```python
from build123d import *

# Parameters (mm, degrees)
F0_R     = 500
F2_DEPTH = 25
F1_R     = 46.69
F3_DEPTH = 300
F4_COUNT = 5


with BuildPart() as f2:
    # F0 (on Top) → F2 (new body)
    with BuildSketch(Plane.XY):
        Circle(F0_R)
    extrude(amount=F2_DEPTH)

    # F1 (on face) → F3 (join)
    with BuildSketch(Plane.XY):
        with Locations((0, -403.2496213913)):
            Circle(F1_R)
    extrude(amount=-F3_DEPTH)

    # F4: F2 ×5 about axis
    f4_axis = Axis((0, 0, 0), (0, 0, 1))


with BuildPart() as f2_1:
    add(f2.part)
    for i in range(1, F4_COUNT):
        add(f2.part.rotate(f4_axis, i * 360 / F4_COUNT))


solid = f2_1.part
```
Work out the finished part from the listing and answer in its coordinate system (mm). A direction names the side the tool comes from. Round coordinates to 2 decimals unless told otherwise and drop trailing zeros. Write each loop counter-clockwise with the first axis right and the second up, starting at its lowest first coordinate (ties: lowest second). Pieces come first, ordered by that corner, then holes.
1) A cutting plane is placed at A-A on x = 0. Determine the outline of the cut face in (y, z).
2) A cutting plane is placed at D-D on x = -219.5. Determine the outline of the cut face in (y, z).
3) Flat-ended cylindrical pins translate along their axes: P1, Ø12, axis at y = -90.5, z = -157, coming from the +X side; P2, Ø5, axis at x = -304, y = 112, coming from the -Z side; P3, Ø10, axis at x = -204.5, z = -213.5, coming from the +Y side. Find the tip coordinate at first contact, or state that the pin passes through.
4) A cutting plane is placed at B-B on z = -151. Determine the outline of the cut face in (x, y), and give its area (3 significant figures).
5) Which of the six approach directions +Z, -Z, +X, -X, +Y, -Y give full straight-line access (tool end or side, diameter ignored) to faces 5 (the face through (-7, 7, 0)), 6 (the face through (-236, 326, -300))?
6) A cutting plane is placed at C-C on y = 0. Determine the outline of the cut face in (x, z), and give its area (3 significant figures).
7) Consider probe 1 along Z at (x, y) = (198, -176.5); probe 2 along X at (y, z) = (-99.5, -115.5); probe 3 along X at (y, z) = (368, -97). Determine where each line is inside the solid, lowest interval first.
8) Determine the mould class of faces 1 (the face through (-383, -124, -300)), 2 (the face through (214.731, 285.212, -147.9)), 3 (the face through (383.937, -77.923, -147.9)), 4 (the face through (21.545, -444.672, -147.9)) for opening direction X: pulls with the +X half, pulls with the -X half, needs draft (parallel to the pull), parting line crosses it, or undercut.
Entries:
1. outline: (-500, 0) - (-449.94, 0) - (-449.94, -300) - (-356.56, -300) - (-356.56, 0) - (500, 0) - (500, 25) - (-500, 25) - close
2. outline: (-449.24, 0) - (282.96, 0) - (282.96, -300) - (369.51, -300) - (369.51, 0) - (449.24, 0) - (449.24, 25) - (-449.24, 25) - close
3. P1: stops at x = 420.79
3. P2: stops at z = 0
3. P3: stops at y = 363.95
4. outline: circle Ø93.38 at (-383.51, -124.61); circle Ø93.38 at (-237.02, 326.24); circle Ø93.38 at (0, -403.25); circle Ø93.38 at (237.02, 326.24); circle Ø93.38 at (383.51, -124.61)
4. area: 34,200 mm2
5. face 5: -Z
5. face 6: -Z, +X, -X, +Y, -Y
6. outline: (-500, 0) - (500, 0) - (500, 25) - (-500, 25) - close
6. area: 25,000 mm2
7. probe 1: z = 0 to 25
7. probe 2: x = -422.88 to -344.15, 344.15 to 422.88
7. probe 3: x = -257.9 to -216.15, 216.15 to 257.9
8. face 1: needs draft
8. face 2: undercut
8. face 3: undercut
8. face 4: parting line crosses it
